Autodesk Inventor part; units mm, degrees
ref_plane "Work Plane1" through (8.6463, -1.4118, -16.3) normal (0, 0, 1) x (1, 0, 0)
ref_plane "Work Plane2" through (8.6463, -39.9118, -14.3) normal (0, 0, 1) x (1, 0, 0)
ref_plane "YZ Plane" through (0, 0, 0) normal (1, 0, 0) x (0, 1, 0)
sketch "Sketch1" plane through (0, 0, 0) normal (0, 0, 1) x (1, 0, 0)
  line L0 (8.6463, -3.6882) -> (-2.6463, -3.6882) construction
  line L1 (8.6463, 3.6882) -> (8.6463, -3.6882) construction
  line L2 (-2.6463, 3.6882) -> (8.6463, 3.6882) construction
  circle A0 centre (5.1537, -0.6118) radius 1.4 construction
  line L3 (-2.6463, -39.9118) -> (8.6463, -39.9118) construction
  line L4 (8.6463, -39.9118) -> (8.6463, -32.5353) construction
  line L5 (8.6463, -32.5353) -> (-2.6463, -32.5353) construction
  circle A1 centre (5.1537, -35.6118) radius 1.4 construction
  line L6 (8.6463, -35.0118) -> (8.6463, -39.9118) construction
  line L7 (8.6463, -39.9118) -> (25.0537, -39.9118) construction
  line L8 (74.7537, -39.9118) -> (74.7537, -34.8118) construction
  line L9 (74.7537, -34.8118) -> (70.7537, -34.8118) construction
  line L10 (70.7537, -34.8118) -> (70.7537, -35.0118) construction
  line L11 (23.2537, -35.0118) -> (8.6463, -35.0118) construction
  line L12 (8.6463, 3.6882) -> (8.6463, -1.2118) construction
  line L13 (8.6463, -1.2118) -> (23.2537, -1.2118) construction
  line L14 (70.7537, -1.2118) -> (70.7537, -1.4118) construction
  line L15 (70.7537, -1.4118) -> (74.7537, -1.4118) construction
  line L16 (74.7537, -1.4118) -> (74.7537, 3.6882) construction
  line L17 (25.0537, 3.6882) -> (8.6463, 3.6882) construction
  line L18 (19.9537, -11.1118) -> (9.9537, -11.1118) construction
  line L19 (9.9537, -16.4118) -> (9.9537, -11.1118) construction
  line L20 (19.9537, -16.4118) -> (9.9537, -16.4118) construction
  line L21 (19.9537, -16.4118) -> (19.9537, -11.1118) construction
  line L22 (-2.6463, 3.6882) -> (22.4609, 3.6882)
  line L23 (22.4609, 3.6882) -> (22.4609, -39.9118)
  line L24 (22.4609, -39.9118) -> (-2.6463, -39.9118)
  line L25 (-2.6463, -39.9118) -> (-2.6463, 3.6882)
  circle A2 centre (5.1537, -0.6118) radius 1.5
  circle A3 centre (5.1537, -35.6118) radius 1.5
  line L26 (14.5908, -13.5618) -> (14.5908, -11.1118) construction
  line L27 (11.6908, -13.5618) -> (11.6908, -11.1118) construction
  line L28 (14.5908, -25.1118) -> (14.5908, -22.6618) construction
  line L29 (11.6908, -25.1118) -> (11.6908, -22.6618) construction
  circle A4 centre (13.1145, -18.1118) radius 2
  line L30 (-2.6463, -32.5353) -> (-2.6463, -39.9118)
  line L31 (34.9537, -32.1118) -> (26.1537, -32.1118)
  line L32 (23.2537, -35.0118) -> (26.1537, -32.1118)
  line L33 (25.0537, -39.9118) -> (25.0537, -39.3319)
  line L34 (26.7161, -37.6695) -> (25.0537, -39.3319)
  arc A5 (27.8115, -36.5741) -> (26.7161, -37.6695) centre (28.2537, -38.1118) ccw
  line L35 (29.4557, -34.9299) -> (27.8115, -36.5741)
  line L36 (36.8518, -34.9299) -> (29.4557, -34.9299)
  line L37 (38.496, -36.5741) -> (36.8518, -34.9299)
  arc A6 (39.5914, -37.6695) -> (38.496, -36.5741) centre (38.0537, -38.1118) ccw
  line L38 (41.2537, -39.3319) -> (39.5914, -37.6695)
  line L39 (41.2537, -39.3319) -> (41.2537, -39.9118)
  line L40 (41.2537, -39.9118) -> (74.7537, -39.9118)
  line L41 (70.7537, -35.0118) -> (44.2537, -35.0118)
  line L42 (41.2537, -32.0118) -> (44.2537, -35.0118)
  line L43 (34.9537, -32.0118) -> (41.2537, -32.0118)
  line L44 (34.9537, -32.0118) -> (34.9537, -32.1118)
  line L45 (34.9537, -4.1118) -> (34.9537, -4.2118)
  line L46 (34.9537, -4.2118) -> (41.2537, -4.2118)
  line L47 (41.2537, -4.2118) -> (44.2537, -1.2118)
  line L48 (44.2537, -1.2118) -> (70.7537, -1.2118)
  line L49 (74.7537, 3.6882) -> (41.2537, 3.6882)
  line L50 (41.2537, 3.6882) -> (41.2537, 3.1083)
  line L51 (41.2537, 3.1083) -> (39.5914, 1.446)
  arc A7 (38.496, 0.3506) -> (39.5914, 1.446) centre (38.0537, 1.8882) ccw
  line L52 (38.496, 0.3506) -> (36.8518, -1.2936)
  line L53 (36.8518, -1.2936) -> (29.4557, -1.2936)
  line L54 (29.4557, -1.2936) -> (27.8115, 0.3506)
  arc A8 (26.7161, 1.446) -> (27.8115, 0.3506) centre (28.2537, 1.8882) ccw
  line L55 (26.7161, 1.446) -> (25.0537, 3.1083)
  line L56 (25.0537, 3.1083) -> (25.0537, 3.6882)
  line L57 (23.2537, -1.2118) -> (26.1537, -4.1118)
  line L58 (26.1537, -4.1118) -> (34.9537, -4.1118)
  line L59 (-2.6463, 3.6882) -> (-2.6463, -3.6882)
  point P0 (0, 0)
  dimension "d0" = 0.1
  dimension "d1" = 0.1
  dimension "d2" = 4
extrude "Extrusion1" add sketch "Sketch1" along normal blind 2
sketch "Sketch2" plane through (0, 0, 0) normal (0, 0, -1) x (-1, 0, 0)
  circle A0 centre (-13.1145, -18.1118) radius 2 construction
  circle A1 centre (-5.1537, -35.6118) radius 1.5 construction
  circle A2 centre (-5.1537, -0.6118) radius 1.5 construction
  line L0 (2.6463, 3.6882) -> (-22.4609, 3.6882) construction
  line L1 (-22.4609, 3.6882) -> (-22.4609, -39.9118) construction
  line L2 (-22.4609, -39.9118) -> (2.6463, -39.9118) construction
  line L3 (2.6463, -39.9118) -> (2.6463, 3.6882) construction
  line L4 (-8.6463, 3.6882) -> (-8.6463, -3.6882) construction
  line L5 (-8.6463, -39.9118) -> (-8.6463, -32.5353) construction
  line L6 (-8.6463, -1.2118) -> (-23.2537, -1.2118) construction
  line L7 (-8.6463, -35.0118) -> (-23.2537, -35.0118) construction
  line L8 (-22.4609, -39.9118) -> (-8.6463, -39.9118)
  line L9 (-8.6463, -39.9118) -> (-8.6463, -35.0118)
  line L10 (-8.6463, -35.0118) -> (-22.4609, -35.0118)
  line L11 (-22.4609, -35.0118) -> (-22.4609, -39.9118)
  line L12 (-22.4609, -39.9118) -> (-22.4609, 3.6882)
  line L13 (-22.4609, -1.2118) -> (-8.6463, -1.2118)
  line L14 (-8.6463, -1.2118) -> (-8.6463, 3.6882)
  line L15 (-8.6463, 3.6882) -> (-22.4609, 3.6882)
  line L16 (-22.4609, 3.6882) -> (-22.4609, -1.2118)
  point P0 (0, 0)
ref_plane "Work Plane1" through (8.6463, -1.4118, -16.3) normal (0, 0, 1) x (1, 0, 0)
ref_plane "Work Plane2" through (8.6463, -39.9118, -14.3) normal (0, 0, 1) x (1, 0, 0)
extrude "Extrusion2" add sketch "Sketch2" along normal up to surface (14.3 mm away)
properties part number "20_focus_inlet_plate_bottom"
Input: part model. Units: mm. Frame: model coordinates. A direction names the side the tool comes from. Round coordinates to 2 decimals unless told otherwise and drop trailing zeros. Loops run counter-clockwise (first coordinate to the right, second up) from the corner with the lowest first, then second, coordinate; pieces in that order, holes last. Notation, with made-up numbers: (-19, 51.25) -> (-11, 51.25) arc R3 cw to (-11, 55.25) -> close; hole circle Ø2 at (0, 25.5). An arc over 180 degrees is marked (long way). One line per item, written item: value.
(1) Material intervals for line 1 (Y direction, x = 14, z = -10.25); line 2 (Z direction, x = 14.5, y = -6); line 3 (X direction, y = -36.5, z = -2.5), sorted ascending. Write a range as [from, to].
Geometry check:
line 1: [-39.91, -35.01], [-1.21, 3.69]
line 2: [0, 2]
line 3: [8.65, 22.46]
(2) Mould query, pull axis X, two halves, no side actions, for faces 1 (the face through (-2.646, -18, 1)), 2 (the face through (22.461, -18, 0.5)), 3 (the face through (15, 3.688, -6)), 4 (the face through (11.53, -16.89, 0.99)). Classes: pulls with the +X half, pulls with the -X half, needs draft (parallel to the pull), parting line crosses it, or undercut.
Geometry check:
face 1: pulls with the -X half
face 2: pulls with the +X half
face 3: needs draft
face 4: undercut
(3) Set-up query: faces 5 (the face through (8.646, 1, -7)), 6 (the face through (10, -18, 2)), 7 (the face through (16, -1.212, -7)). Return all of +Z, -Z, +X, -X, +Y, -Y with unobstructed straight access to the full face (end or side cutting, diameter ignored); none if empty.
Geometry check:
face 5: -Z, -X, +Y, -Y
face 6: +Z, +X, -X, +Y, -Y
face 7: -Z, +X, -X
(4) Section D-D (y = -4). Return the cut outline in (x, z), plus the area to 3 significant figures.
Geometry check:
outline: (-2.65, 0) -> (22.46, 0) -> (22.46, 2) -> (-2.65, 2) -> close
area: 50.2 mm2
(5) Pin query (flat end, axial travel): pin 1 (8 mm diameter, centred on y = -6, z = -4.5, fed in from -X); pin 2 (2 mm diameter, centred on x = 12.5, y = -3, fed in from -Z); pin 3 (1.5 mm diameter, centred on y = 1.5, z = -8, fed in from -X). Return the tip coordinate at first contact, or that it passes through.
Geometry check:
pin 1: through
pin 2: z = 0
pin 3: x = 8.65
(6) Section B-B (x = 17.25). Return the cut outline in (y, z).
Geometry check:
outline: (-39.91, -14.3) -> (-35.01, -14.3) -> (-35.01, 0) -> (-1.21, 0) -> (-1.21, -14.3) -> (3.69, -14.3) -> (3.69, 2) -> (-39.91, 2) -> close
(7) Section C-C (x = 4.75). Return the cut outline in (y, z).
Geometry check:
outline: (-39.91, 0) -> (-37.06, 0) -> (-37.06, 2) -> (-39.91, 2) -> close; (-34.17, 0) -> (-2.06, 0) -> (-2.06, 2) -> (-34.17, 2) -> close; (0.83, 0) -> (3.69, 0) -> (3.69, 2) -> (0.83, 2) -> close
(8) Section A-A (z = -8.25). Return the cut outline in (x, y).
Geometry check:
outline: (8.65, -39.91) -> (22.46, -39.91) -> (22.46, -35.01) -> (8.65, -35.01) -> close; (8.65, -1.21) -> (22.46, -1.21) -> (22.46, 3.69) -> (8.65, 3.69) -> close
